Input: part model. Units: mm. Frame: model coordinates. A direction names the side the tool comes from. Give positions to 0.01 mm unless a question says otherwise; leave off trailing zeros. Order: outer loops, then holes, each group sorted by start corner. A loop starts at its lowest first (then second) coordinate and runs counter-clockwise, first axis right, second up.
```python
from build123d import *

# Parameters (mm, degrees)
PAD_DEPTH       = 20
SKETCH001_R     = 1.6
POCKET_DEPTH    = 6
SKETCH002_R     = 4
POCKET001_DEPTH = 117.001
FILLET_R        = 4
FILLET001_R     = 4
FILLET002_R     = 4
FILLET003_R     = 3


with BuildPart() as part:
    # Sketch → Pad (new body)
    with BuildSketch(Plane.XY):
        Polygon((38.5, 0), (-38.5, 0), (-38.5, 20), (-58.5, 20), (-58.5, 86), (-52.5, 86), (-52.5, 26), (-32.5, 26), (-32.5, 6), (32.5, 6), (32.5, 26), (52.5, 26), (52.5, 86), (58.5, 86), (58.5, 20), (38.5, 20), align=None)
    extrude(amount=PAD_DEPTH)

    # Sketch001 (on Face9 of Pad) → Pocket (cut)
    with BuildSketch(Plane(origin=(0, 6, 0), x_dir=(-1, 0, 0), z_dir=(0, 1, 0))):
        with Locations((-25, 15)):
            Circle(SKETCH001_R)
        with Locations((-25, 5)):
            Circle(SKETCH001_R)
        with Locations((25, 15)):
            Circle(SKETCH001_R)
        with Locations((25, 5)):
            Circle(SKETCH001_R)
    extrude(amount=-POCKET_DEPTH, mode=Mode.SUBTRACT)

    # Sketch002 (on Face22 of Pocket) → Pocket001 (cut, through all)
    with BuildSketch(Plane.YZ.offset(58.5)):
        with Locations((78.5, 10)):
            Circle(SKETCH002_R)
    extrude(amount=-POCKET001_DEPTH, mode=Mode.SUBTRACT)

    # Fillet
    fillet_edges = [part.edges().sort_by_distance(p)[0] for p in [
        (-32.5, 6, 10),
        (52.5, 26, 10),
        (32.5, 6, 10),
        (-52.5, 26, 10),
    ]]
    fillet(fillet_edges, radius=FILLET_R)

    # Fillet001
    fillet001_edges = [part.edges().sort_by_distance(p)[0] for p in [
        (32.5, 26, 10),
        (-32.5, 26, 10),
        (-58.5, 20, 10),
        (-38.5, 0, 10),
        (58.5, 20, 10),
        (38.5, 0, 10),
    ]]
    fillet(fillet001_edges, radius=FILLET001_R)

    # Fillet002
    fillet002_edges = [part.edges().sort_by_distance(p)[0] for p in [
        (38.5, 20, 10),
        (-38.5, 20, 10),
    ]]
    fillet(fillet002_edges, radius=FILLET002_R)

    # Fillet003
    fillet003_edges = [part.edges().sort_by_distance(p)[0] for p in [
        (55.5, 86, 0),
        (-55.5, 86, 0),
        (55.5, 86, 20),
        (-55.5, 86, 20),
    ]]
    fillet(fillet003_edges, radius=FILLET003_R)


solid = part.part
```
1) Cut plane D-D (z = 10). Count the separate pieces of the cut face and the enclosed holes in it, then the cut area to 3 significant figures.
2) Cut plane C-C (y = 78.5). Return the cut outline in (x, z), then the cut area to 3 significant figures.
3) Cut plane A-A (y = 68). Return the cut outline in (x, z).
4) Pull-direction query (Z, two-part tool) for faces 1 (the face through (-23.82, 3.04, 16.08)), 2 (the face through (55, 86, 10)), 3 (the face through (55.54, 85.14, 19.1)); classes: pulls with the +Z half, pulls with the -Z half, needs draft (parallel to the pull), parting line crosses it, or undercut.
5) Line query: probe 1 along X at (y, z) = (52, 6); probe 2 along Z at (x, y) = (-55.3, 78.5); probe 3 along Z at (x, y) = (-25, 2.9). Output: solid intervals per line, ascending.
6) Cut plane B-B (x = -25). Return the cut outline in (y, z).
7) First-contact query: P1, Ø6, axis at x = -48.5, z = 11, coming from the -Y side; P2, Ø1.9, axis at x = -25, z = 5, coming from the +Y side; P3, Ø3.5, axis at x = 40.5, z = 14.5, coming from the +Y side; P4, Ø10, axis at x = 17, z = 3.5, coming from the +Y side. Flat tips, straight axial feed; report the tip coordinate or a pass-through.
8) Reachability of faces 4 (the face through (49, 20, 10)), 5 (the face through (-48, 20, 10)), 6 (the face through (0, 5, 0)), 7 (the face through (0, 6, 10)) from +Z, -Z, +X, -X, +Y, -Y: full face, straight path, thin tool, end or side. Return the list, or none.
Geometry says:
1. separate pieces: 3
1. enclosed holes: 0
1. area: 1,570 mm2
2. outline: (-58.5, 0) - (-52.5, 0) - (-52.5, 6) - (-58.5, 6) - close; (-58.5, 14) - (-52.5, 14) - (-52.5, 20) - (-58.5, 20) - close; (52.5, 0) - (58.5, 0) - (58.5, 6) - (52.5, 6) - close; (52.5, 14) - (58.5, 14) - (58.5, 20) - (52.5, 20) - close
2. area: 144 mm2
3. outline: (-58.5, 0) - (-52.5, 0) - (-52.5, 20) - (-58.5, 20) - close; (52.5, 0) - (58.5, 0) - (58.5, 20) - (52.5, 20) - close
4. face 1: undercut
4. face 2: needs draft
4. face 3: pulls with the +Z half
5. probe 1: x = -58.5 to -52.5, 52.5 to 58.5
5. probe 2: z = 0 to 6, 14 to 20
5. probe 3: z = 0 to 3.4, 6.6 to 13.4, 16.6 to 20
6. outline: (0, 0) - (6, 0) - (6, 3.4) - (0, 3.4) - close; (0, 6.6) - (6, 6.6) - (6, 13.4) - (0, 13.4) - close; (0, 16.6) - (6, 16.6) - (6, 20) - (0, 20) - close
7. P1: stops at y = 20
7. P2: passes through
7. P3: stops at y = 26
7. P4: stops at y = 6
8. face 4: +Z, -Z, +X, -Y
8. face 5: +Z, -Z, -X, -Y
8. face 6: -Z, +X, -X, +Y, -Y
8. face 7: +Z, -Z, +Y
